Can you work these out from the model? Positions are in its coordinate system, mm. A direction names the side the tool comes from. Coordinates: 2 decimals unless noted, no trailing zeros. Order: outer loops, then holes, each group sorted by start corner. A loop starts at its lowest first (then second) coordinate and runs counter-clockwise, first axis right, second up. Notation, with made-up numbers: (56, 74) - (105, 74) arc R30 ccw to (105, 108) - close; hole circle Ø2 at (87, -4). An arc over 180 degrees is marked (long way). Use a Markdown table: item, result. Add a question column.
(1) For pin 1 Ø2.5 at (x, y) = (7.5, 7) entering from -Z; pin 2 Ø1.5 at (x, y) = (10.5, -4.5) entering from +Z; pin 3 Ø1.2 at (x, z) = (12.5, 8) entering from -Y; pin 4 Ø7.5 at (y, z) = (-6, 3) entering from +X, each with a flat end and sliding along its axis, tell me the tip position at first contact or that it passes through.
(2) On a 3-axis mill with a long thin cutter (end or side, diameter ignored), from which of +Z, -Z, +X, -X, +Y, -Y can I reach the whole of each face in a straight line? I mean faces 1 (the flat face through (14, -3.5, 9)), 2 (the flat face through (6, 7.8, 0)), 3 (the flat face through (7, -10, -0.75)), 4 (the cylindrical face through (13.5, -0.1, 6.5)), 5 (the flat face through (14, 3.5, -9)). Say none if no direction works.
(3) I want a section at C-C (z = 4). State how many separate pieces and enclosed holes the cut face has, and give its area (3 significant figures).
(4) If I drill on L1, parallel to X at y = -8.4, z = -1.85; L2, parallel to X at y = -8.4, z = 6.5; L3, parallel to Z at x = 10, y = -2.5, over which ranges is the centre line in solid material (lowest first)? Write a range as [from, to].
(5) I want a section at B-B (x = 5). List the corners of the cut face in (y, z) for me, and give its area (3 significant figures).
(6) We'd pull the mould along Z, two halves only. Please class faces 6 (the flat face through (3, -10, -5)), 7 (the flat face through (15.5, 0, 9)), 8 (the flat face through (6, 7, -2)): pulls with the +Z half, pulls with the -Z half, needs draft (parallel to the pull), parting line crosses it, or undercut.
(7) I want a section at A-A (y = 0). List the corners of the cut face in (x, z) for me, and give its area (3 significant figures).
Autodesk Inventor part; units mm, degrees
ref_plane "L_XY" through (15.2, 0, 0) normal (1, 0, 0) x (0, 0, -1)
ref_plane "L_YZ" through (15.2, 0, 0) normal (0, 0, -1) x (0, 1, 0)
ref_plane "L_ZX" through (15.2, 0, 0) normal (0, 1, 0) x (1, 0, 0)
sketch "Sketch_1" plane through (0, 0, 0) normal (0, 0, 1) x (1, 0, 0)
  line L0 (15.5, 0) -> (0, 0)
  line L1 (0, 0) -> (0, 12.8)
  line L2 (0, 12.8) -> (0.2, 13)
  line L3 (0.2, 13) -> (15.5, 13)
  line L4 (15.5, 13) -> (15.5, 0)
  line L5 (15.5, 0) -> (0, 0)
revolve "Revolution1" add sketch "Sketch_1" angle 360 about axis through (15.5, 0, 0) along (1, 0, 0)
sketch "Sketch_6" plane through (0, 0, 0) normal (1, 0, 0) x (0, 1, 0)
  line L0 (-13, 0.75) -> (-13, -0.75)
  line L1 (-13, -0.75) -> (0, -0.75)
  line L2 (0, -0.75) -> (0, 0.75)
  line L3 (0, 0.75) -> (-13, 0.75)
extrude "Extrusion1" cut sketch "Sketch_6" along normal blind 11.5
sketch "Sketch_7" plane through (5, 0, 0) normal (1, 0, 0) x (0, 0, -1)
  line L0 (-13, -8.4) -> (13, -8.4)
  line L1 (13, -8.4) -> (13, -11.9)
  line L2 (13, -11.9) -> (5, -11.9)
  line L3 (5, -11.9) -> (5, -10.4)
  line L4 (5, -10.4) -> (0.75, -10.4)
  line L5 (0.75, -10.4) -> (0.75, -8.4)
  line L6 (0.75, -8.4) -> (13, -8.4)
revolve "Revolution2" cut sketch "Sketch_7" angle 360 about axis through (5, -8.4, 13) along (0, 0, 1)
sketch "Sketch4" plane through (11.5, 0, 0.75) normal (0, 0, -1) x (-1, 0, 0)
  point P0 (6.5, -8.4)
hole "Hole1" at (5, -8.4, 0.75) direction (0, 0, 1) diameter 3.242 depth 12.25
sketch "Sketch_2" plane through (15.5, 0, 0) normal (1, 0, 0) x (0, 0, -1)
  line L0 (-14, -13.5) -> (14, -13.5)
  line L1 (14, -13.5) -> (14, 13.5)
  line L2 (14, 13.5) -> (-14, 13.5)
  line L3 (-14, 13.5) -> (-14, -13.5)
  line L4 (-13, -3.5) -> (13, -3.5)
  line L5 (13, -3.5) -> (13, 3.5)
  line L6 (13, 3.5) -> (-13, 3.5)
  line L7 (-13, 3.5) -> (-13, -3.5)
extrude "Extrusion2" cut sketch "Sketch_2" against normal blind 4
sketch "Sketch6" plane through (15.5, 0, 0) normal (1, 0, 0) x (0, 0, -1)
  point P0 (0, 0)
hole "Hole2" at (15.5, 0, 0) direction (-1, 0, 0) diameter 13 depth 4
sketch "Sketch_15" plane through (11.5, 0, 0) normal (1, 0, 0) x (0, 0, -1)
  arc A0 (-2, 5.6569) -> (2, 5.6569) centre (0, 0) ccw
  line L0 (2, 5.6569) -> (2, 7.8)
  line L1 (2, 7.8) -> (-2, 7.8)
  line L2 (-2, 7.8) -> (-2, 5.6569)
extrude "Extrusion3" cut sketch "Sketch_15" along normal mid plane 31
ref_plane "L_XY" through (15.2, 0, 0) normal (1, 0, 0) x (0, 0, -1)
ref_plane "L_YZ" through (15.2, 0, 0) normal (0, 0, -1) x (0, 1, 0)
ref_plane "L_ZX" through (15.2, 0, 0) normal (0, 1, 0) x (1, 0, 0)
ref_plane "screw_XY" through (5, -8.4, -5) normal (0, 0, -1) x (1, 0, 0)
ref_plane "screw_YZ" through (5, -8.4, -5) normal (1, 0, 0) x (0, -1, 0)
ref_plane "screw_ZX" through (5, -8.4, -5) normal (0, -1, 0) x (0, 0, -1)
properties part number "MCOCWK26-12_c"
Answers follow:
| question | item | result |
|---|---|---|
| 1 | pin 1 | stops at z = -11.66 |
| 1 | pin 2 | stops at z = 12.45 |
| 1 | pin 3 | stops at y = -3.5 |
| 1 | pin 4 | stops at x = 15.5 |
| 2 | face 1 | +Z, -Z, +X, -Y |
| 2 | face 2 | +X, -X |
| 2 | face 3 | +X, -X, -Y |
| 2 | face 4 | +X |
| 2 | face 5 | +Z, -Z, +X, +Y |
| 3 | separate pieces | 2 |
| 3 | enclosed holes | 1 |
| 3 | area | 173 mm² |
| 4 | L1 | x = [0, 3], [7, 11.5] |
| 4 | L2 | x = [0, 3.38], [6.62, 11.5] |
| 4 | L3 | z = [-12.76, -5.45], [5.45, 12.76] |
| 5 | outline | (-12.98, -0.75) arc R13 ccw to (-11.9, -5.23) - (-11.9, -5) - (-10.4, -5) - (-10.4, -0.75) - close; (-12.98, 0.75) - (-10.02, 0.75) - (-10.02, 8.28) arc R13 ccw to start; (-6.78, 0.75) - (-5.95, 0.75) arc R6 cw to (5.66, 2) - (7.8, 2) - (7.8, -2) - (5.66, -2) arc R6 cw to (-5.95, -0.75) - (-6.4, -0.75) - (-6.4, -5) - (-4.9, -5) - (-4.9, -12.04) arc R13 ccw (long way) to (-6.78, 11.09) - close |
| 5 | area | 321 mm² |
| 6 | face 6 | pulls with the -Z half |
| 6 | face 7 | needs draft |
| 6 | face 8 | undercut |
| 7 | outline | (0, -12.8) - (0.2, -13) - (15.5, -13) - (15.5, -6.5) - (11.5, -6.5) - (11.5, -6) - (0, -6) - close; (0, 6) - (11.5, 6) - (11.5, 6.5) - (15.5, 6.5) - (15.5, 13) - (0.2, 13) - (0, 12.8) - close |
| 7 | area | 213 mm² |
